```python
from build123d import *

# Parameters (mm, degrees)
F0_W     = 100
F0_H     = 50
F0_W_2   = 94
F0_H_2   = 44
F1_DEPTH = 1000
F2_W     = 200
F2_H     = 100
F3_DEPTH = 10
F4_R     = 6
F5_DEPTH = 25
F6_R     = 5
F7_R     = 8
F8_DEPTH = 50


with BuildPart() as f1:
    # F0 (on Top) → F1 (new body)
    with BuildSketch(Plane.XY):
        Rectangle(F0_W, F0_H)
        Rectangle(F0_W_2, F0_H_2, mode=Mode.SUBTRACT)
    extrude(amount=F1_DEPTH)

    # F2 (on Top) → F3 (join)
    with BuildSketch(Plane.XY):
        Rectangle(F2_W, F2_H)
    extrude(amount=-F3_DEPTH)

    # F4 (on face) → F5 (cut)
    with BuildSketch(Plane(origin=(0, 0, -10), x_dir=(1, 0, 0), z_dir=(0, 0, -1))):
        with Locations((-80, 35)):
            Circle(F4_R)
        with Locations((-80, -35)):
            Circle(F4_R)
        with Locations((80, 35)):
            Circle(F4_R)
        with Locations((80, -35)):
            Circle(F4_R)
    extrude(amount=-F5_DEPTH, mode=Mode.SUBTRACT)

    # F6
    f6_edges = [f1.edges().sort_by_distance(p)[0] for p in [
        (100, -50, -5),
        (100, 50, -5),
        (-100, -50, -5),
        (-100, 50, -5),
    ]]
    fillet(f6_edges, radius=F6_R)

    # F7 (on face) → F8 (cut)
    with BuildSketch(Plane.XZ.offset(25)):
        with Locations((-30, 988)):
            Circle(F7_R)
        with Locations((30, 988)):
            Circle(F7_R)
        with Locations((30, 962)):
            Circle(F7_R)
        with Locations((-30, 962)):
            Circle(F7_R)
    extrude(amount=-F8_DEPTH, mode=Mode.SUBTRACT)


solid = f1.part
```
Read the model definition and answer for the solid it produces. Units are mm, in the model's axes. A direction names the side the tool comes from. Coordinates: 2 decimals unless noted, no trailing zeros. Write each loop counter-clockwise with the first axis right and the second up, starting at its lowest first coordinate (ties: lowest second). Pieces come first, ordered by that corner, then holes. Notation, with made-up numbers: (89.25, 69) -> (139.25, 69) arc R18 cw to (139.25, 90) -> close; hole circle Ø8 at (-8, -21.5). An arc over 180 degrees is marked (long way). Write item = value, one per line.
(1) Which of the six approach directions +Z, -Z, +X, -X, +Y, -Y give full straight-line access (tool end or side, diameter ignored) to faces 1 (the face through (50, 0, 493)), 2 (the face through (-50, 0, 493)), 3 (the face through (-1, 25, 493)), 4 (the face through (-1, 0, 0))?
From the geometry:
face_1 = +Z, +X, +Y, -Y
face_2 = +Z, -X, +Y, -Y
face_3 = +Z, +X, -X, +Y
face_4 = +Z
(2) Straight lines are drawn through the part: L1, parallel to Y at x = -80, z = -4.75; L2, parallel to X at y = -35, z = -4.75; L3, parallel to X at y = 24, z = 962. For each, find the intervals that lie inside material, in ascending order. Write a range as from..to.
From the geometry:
L1 = -50..-41, -29..29, 41..50
L2 = -100..-86, -74..74, 86..100
L3 = -50..-38, -22..22, 38..50
(3) Given pin 1 Ø9.5 at (x, z) = (30, 988) entering from +Y; pin 2 Ø25 at (y, z) = (9, 551.5) entering from +X; pin 3 Ø3 at (x, y) = (21.5, -38) entering from +Z; pin 4 Ø1.5 at (x, z) = (48.5, 192) entering from +Y, each flat-ended and moving along its own axis, determine where each tip first touches the part or whether it passes through.
From the geometry:
pin_1 = through
pin_2 = 50
pin_3 = 0
pin_4 = 25
(4) Section A-A on z = 722 is taken. Write down the section's boundary in (x, y), plus the area to 3 significant figures.
From the geometry:
outline = (-50, -25) -> (50, -25) -> (50, 25) -> (-50, 25) -> close; hole (-47, -22) -> (47, -22) -> (47, 22) -> (-47, 22) -> close
area = 864 mm2
(5) For a pull along Y with two mould halves and no side action, classify faces 5 (the face through (47, 0, 493)), 6 (the face through (33.69, 23.48, 954.9)), 7 (the face through (-1, -25, 493)) as +Y half, -Y half, draft (parallel to the pull), parting line (faces both ways), or undercut.
From the geometry:
face_5 = undercut
face_6 = draft
face_7 = -Y half
(6) Section B-B on y = -8.5 is taken. Write down the section's boundary in (x, z).
From the geometry:
outline = (-100, -10) -> (100, -10) -> (100, 0) -> (50, 0) -> (50, 1000) -> (47, 1000) -> (47, 0) -> (-47, 0) -> (-47, 1000) -> (-50, 1000) -> (-50, 0) -> (-100, 0) -> close
